from build123d import *

# Parameters (mm, degrees)
CROQUIS2_R            = 3.95
CORTAR_EXTRUIR1_DEPTH = 14
CROQUIS3_R            = 10.95
CORTAR_EXTRUIR2_DEPTH = 115.8
CROQUIS4_R            = 2.5
CORTAR_EXTRUIR3_DEPTH = 43


with BuildPart() as part:
    # Croquis1 → Revolución1 (revolve)
    with BuildSketch(Plane.XY, mode=Mode.PRIVATE) as revoluci_n1_sk:
        with BuildLine():
            Line((5.952239129, 4.74561549), (2.952239129, -1.25438451))
            ThreePointArc((2.952239129, -1.25438451), (0.452239129, -2.455946629), (-2.047760871, -1.25438451))
            Line((-2.047760871, -1.25438451), (-5.047760871, 4.74561549))
            Line((-5.047760871, 4.74561549), (-7.047760871, 4.74561549))
            Line((-7.047760871, 4.74561549), (-7.047760871, -20.25438451))
            Line((-7.047760871, -20.25438451), (7.952239129, -20.25438451))
            Line((7.952239129, -20.25438451), (7.952239129, 4.74561549))
            Line((7.952239129, 4.74561549), (5.952239129, 4.74561549))
        make_face()
    revolve(revoluci_n1_sk.sketch.rotate(Axis((-20.844407183, -20.25438451, 0), (1, 0, 0)), 90), axis=Axis((-20.844407183, -20.25438451, 0), (1, 0, 0)))

    # Croquis2 → Cortar-Extruir1 (cut)
    with BuildSketch(Plane.ZY.offset(7.047760871)):
        with Locations((0, -20.25438451)):
            Circle(CROQUIS2_R)
    extrude(amount=-CORTAR_EXTRUIR1_DEPTH, mode=Mode.SUBTRACT)

    # Croquis3 → Cortar-Extruir2 (cut)
    with BuildSketch(Plane.ZY.offset(7.047760871)):
        with Locations((0, -20.25438451)):
            Circle(CROQUIS3_R)
    extrude(amount=-CORTAR_EXTRUIR2_DEPTH, mode=Mode.SUBTRACT)

    # Croquis4 → Cortar-Extruir3 (cut)
    with BuildSketch(Plane(origin=(7.952239129, 0, 0), x_dir=(0, 0, -1), z_dir=(1, 0, 0))):
        with Locations((-15, -20.25438451)):
            Circle(CROQUIS4_R)
        with Locations((0, -35.25438451)):
            Circle(CROQUIS4_R)
        with Locations((15, -20.25438451)):
            Circle(CROQUIS4_R)
        with Locations((0, -5.25438451)):
            Circle(CROQUIS4_R)
    extrude(amount=-CORTAR_EXTRUIR3_DEPTH, mode=Mode.SUBTRACT)


solid = part.part
Read the model definition and answer for the solid it produces. Units are mm, in the model's axes. A direction names the side the tool comes from. Round coordinates to 2 decimals unless told otherwise and drop trailing zeros. Write each loop counter-clockwise with the first axis right and the second up, starting at its lowest first coordinate (ties: lowest second). Pieces come first, ordered by that corner, then holes.
1. The part is cut by section B-B, the plane x = -4.25. Determine the outline of the cut face in (y, z).
2. The part is cut by section A-A, the plane z = 0. Determine the outline of the cut face in (x, y), then the cut area to 3 significant figures.
3. Straight lines are drawn through the part: L1, parallel to Z at x = 7, y = -19; L2, parallel to Y at x = 2.5, z = 0; L3, parallel to X at y = -36, z = 12. For each, find the intervals that lie inside material, in ascending order.
4. Given pin 1 Ø5 at (x, y) = (-5, -13.5) entering from -Z; pin 2 Ø5 at (x, z) = (-5.5, 8) entering from +Y; pin 3 Ø2 at (x, y) = (-0.5, -11) entering from +Z, each flat-ended and moving along its own axis, determine where each tip first touches the part or whether it passes through.
5. Determine the mould class of faces 1 (the face through (0.35, -9.4, -1.43)), 2 (the face through (-7.048, -9, 5)), 3 (the face through (3.1, -1.42, -4.18)) for opening direction Z: pulls with the +Z half, pulls with the -Z half, needs draft (parallel to the pull), parting line crosses it, or undercut.
6. Which of the six approach directions +Z, -Z, +X, -X, +Y, -Y give full straight-line access (tool end or side, diameter ignored) to faces 4 (the face through (6.938, 1.925, 11.536)), 5 (the face through (-2.235, -3.065, 8.941))?
Values:
1. outline: circle Ø46.81 at (-20.25, 0); hole circle Ø5 at (-35.25, 0); hole circle Ø21.9 at (-20.25, 0); hole circle Ø5 at (-20.25, -15); hole circle Ø5 at (-20.25, 15); hole circle Ø5 at (-5.25, 0)
2. outline: (-7.05, -45.25) - (-5.05, -45.25) - (-2.05, -39.25) arc R3.2 cw to (2.95, -39.25) - (5.95, -45.25) - (7.95, -45.25) - (7.95, -37.75) - (-7.05, -37.75) - close; (-7.05, -32.75) - (7.95, -32.75) - (7.95, -31.2) - (-7.05, -31.2) - close; (-7.05, -9.3) - (7.95, -9.3) - (7.95, -7.75) - (-7.05, -7.75) - close; (-7.05, -2.75) - (7.95, -2.75) - (7.95, 4.75) - (5.95, 4.75) - (2.95, -1.25) arc R3.2 cw to (-2.05, -1.25) - (-5.05, 4.75) - (-7.05, 4.75) - close
2. area: 167 mm2
3. L1: z = -24.97 to -17.16, -12.84 to -10.88, 10.88 to 12.84, 17.16 to 24.97
3. L2: y = -38.79 to -37.75, -32.75 to -31.2, -9.3 to -7.75, -2.75 to -1.72
3. L3: x = -7.05 to -2.45, 3.35 to 7.95
4. pin 1: stops at z = -24.64
4. pin 2: stops at y = 4.13
4. pin 3: stops at z = 16.15
5. face 1: undercut
5. face 2: needs draft
5. face 3: parting line crosses it
6. face 4: +X, -X
6. face 5: none
